Part model, mm, in its own coordinate system. A direction names the side the tool comes from. Give positions to 0.01 mm unless a question says otherwise; leave off trailing zeros. Order: outer loops, then holes, each group sorted by start corner. A loop starts at its lowest first (then second) coordinate and runs counter-clockwise, first axis right, second up. Notation, with made-up numbers: M 2,81.5 L 50,81.5 A13 ccw 50,88.5 Z; hole C 27,71 d2. An arc over 180 degrees is marked long. Answer as a JSON object with one key per item and string values.
from build123d import *

# Parameters (mm, degrees)
BOSS_EXTRUDE1_DEPTH     = 5
SKETCH2_W               = 5.1
SKETCH2_H               = 2.05
CUT_EXTRUDE1_DEPTH      = 1
CUT_EXTRUDE1_DEPTH_BACK = 60.1838596
CUT_EXTRUDE2_REACH      = 116.127
SKETCH3_W               = 10
SKETCH3_H               = 2
SKETCH4_W               = 4.444636185
SKETCH4_H               = 5
BOSS_EXTRUDE2_DEPTH     = 45.135921
SKETCH5_W               = 0.1
SKETCH5_H               = 2
BOSS_EXTRUDE3_DEPTH     = 37.960973


with BuildPart() as part:
    # Sketch1 → Boss-Extrude1 (new body)
    with BuildSketch(Plane(origin=(0, 0, 0), x_dir=(1, 0, 0), z_dir=(0, 1, 0))):
        Polygon((0, 0), (114.126652136, 0), (114.126652136, 45.135921053), (114.126652136, 59.1838596), (76.165679632, 59.1838596), (76.165679632, 45.135921053), (0, 45.135921053), align=None)
    extrude(amount=BOSS_EXTRUDE1_DEPTH)

    # Sketch2 → Cut-Extrude1 (cut, two sides)
    with BuildSketch(Plane.XY) as cut_extrude1_sk:
        with Locations((2.5, 3.975)):
            Rectangle(SKETCH2_W, SKETCH2_H)
        with Locations((52.62, 3.975)):
            Rectangle(SKETCH2_W, SKETCH2_H)
    extrude(amount=CUT_EXTRUDE1_DEPTH, mode=Mode.SUBTRACT)
    extrude(cut_extrude1_sk.sketch, amount=-CUT_EXTRUDE1_DEPTH_BACK, mode=Mode.SUBTRACT)

    # Sketch3 → Cut-Extrude2 (cut, up to next)
    with BuildSketch(Plane(origin=(114.126652136, -2e-09, 0), x_dir=(0, 0, -1), z_dir=(1, 0, 0)), mode=Mode.PRIVATE) as cut_extrude2_sk1:
        with Locations((50.135921053, 4.000000002)):
            Rectangle(SKETCH3_W, SKETCH3_H)
    cut_extrude2_tool1 = extrude(cut_extrude2_sk1.sketch, amount=-CUT_EXTRUDE2_REACH, mode=Mode.PRIVATE) & part.part
    add(cut_extrude2_tool1.solids().sort_by_distance((114.126652, 4, -50.135921))[0], mode=Mode.SUBTRACT)

    # Sketch4 → Boss-Extrude2 (add)
    with BuildSketch(Plane.XY):
        with Locations((-2.222318093, 2.5)):
            Rectangle(SKETCH4_W, SKETCH4_H)
    extrude(amount=-BOSS_EXTRUDE2_DEPTH)

    # Sketch5 → Boss-Extrude3 (add)
    with BuildSketch(Plane(origin=(114.126652136, 0, 0), x_dir=(0, 0, -1), z_dir=(1, 0, 0))):
        with Locations((45.185921053, 4)):
            Rectangle(SKETCH5_W, SKETCH5_H)
    extrude(amount=-BOSS_EXTRUDE3_DEPTH)


solid = part.part
1. Which spindle directions (+Z, -Z, +X, -X, +Y, -Y) get a long thin tool onto all of the face, cutting with end or side? Do faces 1 (the flat face through (55.17, 4, -22)), 2 (the flat face through (27, 5, -23)), 3 (the flat face through (35, 3, -45.136)), 4 (the flat face through (95, 4, -45.236)). Say none if no direction does.
Worked answers:
{"face 1": "+Z, -Z, +Y", "face 2": "+Z, -Z, +X, -X, +Y", "face 3": "-Z, -X, +Y, -Y", "face 4": "+X, -X, +Y"}
2. Cut at A-A on x = 88.5. Give the cut face in (y, z), plus the area to 3 significant figures.
Worked answers:
{"outline": "M 0,-59.18 L 5,-59.18 L 5,-55.14 L 3,-55.14 L 3,-45.24 L 5,-45.24 L 5,0 L 0,0 Z", "area": "276 mm^2"}
3. Cut at C-C on z = -40.5. Give the cut face in (x, y), plus the area to 3 significant figures.
Worked answers:
{"outline": "M -4.44,0 L 114.13,0 L 114.13,5 L 55.17,5 L 55.17,2.95 L 50.07,2.95 L 50.07,5 L 5.05,5 L 5.05,2.95 L 0,2.95 L 0,5 L -4.44,5 Z", "area": "572 mm^2"}
4. Pin check, flat tips, straight feed: P1, Ø2.5, axis at x = 55, y = 3, coming from the -Z side; P2, Ø4, axis at x = 75.5, z = -51, coming from the +Y side. Stop position of each tip, or through.
Worked answers:
{"P1": "stops at z = -45.14", "P2": "stops at y = 3"}
5. Probe line 1 along X through (y, z) = (4.5, -32); line 2 along Z through (x, y) = (61, 0.9); line 3 along Y through (x, z) = (83, -48). List the from-to ranges inside material, lowest first.
Worked answers:
{"line 1": "x = -4.44 to 0, 5.05 to 50.07, 55.17 to 114.13", "line 2": "z = -45.14 to 0", "line 3": "y = 0 to 3"}
6. Cut at B-B on y = 0.8. Give the cut face in (x, z).
Worked answers:
{"outline": "M -4.44,-45.14 L 76.17,-45.14 L 76.17,-59.18 L 114.13,-59.18 L 114.13,0 L -4.44,0 Z"}
7. Cut at D-D on x = 20.5. Give the cut face in (y, z).
Worked answers:
{"outline": "M 0,-45.14 L 5,-45.14 L 5,0 L 0,0 Z"}
8. Two-plate mould, pull along Z, no slides. Class faces 5 (the flat face through (95, 2, -59.184)), 6 (the flat face through (95, 4, -55.136)), 7 (the flat face through (85, 5, -22)): +Z half, -Z half, draft (parallel to the pull), parting line (faces both ways), or undercut.
Worked answers:
{"face 5": "-Z half", "face 6": "undercut", "face 7": "draft"}
